```python
from build123d import *

# Parameters (mm, degrees)
IZIM1_W                     = 112.077867903
IZIM1_H                     = 74.551796061
Y_KSEKLIK_EKSTR_ZYON1_DEPTH = 83.934945503
IZIM2_W                     = 101.231343604
IZIM2_H                     = 66.034767048
KES_EKSTR_ZYON2_DEPTH       = 76.644430763
IZIM3_W                     = 39.444954406
IZIM3_H                     = 29.43714267
KES_EKSTR_ZYON3_DEPTH       = 88.138
Y_KSEKLIK_EKSTR_ZYON2_DEPTH = 2.54


with BuildPart() as part:
    # Çizim1 → Yükseklik-Ekstrüzyon1 (new body)
    with BuildSketch(Plane.XY):
        with Locations((-65.092964498, -0.375260719)):
            Rectangle(IZIM1_W, IZIM1_H)
    extrude(amount=Y_KSEKLIK_EKSTR_ZYON1_DEPTH)

    # Çizim2 → Kes-Ekstrüzyon2 (cut)
    with BuildSketch(Plane.XY.offset(83.934945503)):
        with Locations((-64.892181627, -1.311030391)):
            Rectangle(IZIM2_W, IZIM2_H)
    extrude(amount=-KES_EKSTR_ZYON2_DEPTH, mode=Mode.SUBTRACT)

    # Çizim3 → Kes-Ekstrüzyon3 (cut)
    with BuildSketch(Plane.XY.offset(7.29051474)):
        with Locations((-56.533774773, 7.010455604)):
            Rectangle(IZIM3_W, IZIM3_H)
    extrude(amount=-KES_EKSTR_ZYON3_DEPTH, mode=Mode.SUBTRACT)

    # Çizim4 → Yükseklik-Ekstrüzyon2 (add)
    with BuildSketch(Plane(origin=(0, -37.651158749, 0), x_dir=(-1, 0, 0), z_dir=(0, -1, 0))):
        with BuildLine():
            Line((113.611032553, -79.46460314), (113.611032553, -6.689235104))
            ThreePointArc((113.611032553, -6.689235104), (115.960654564, -4.339613094), (118.310276574, -6.689235104))
            Line((118.310276574, -6.689235104), (118.310276574, -79.46460314))
            ThreePointArc((118.310276574, -79.46460314), (115.960654564, -81.814225151), (113.611032553, -79.46460314))
        make_face()
        with BuildLine():
            Line((11.064518037, -78.985150192), (11.064518037, -6.209782156))
            ThreePointArc((11.064518037, -6.209782156), (13.414140048, -3.860160145), (15.763762058, -6.209782156))
            Line((15.763762058, -6.209782156), (15.763762058, -78.985150192))
            ThreePointArc((15.763762058, -78.985150192), (13.414140048, -81.334772203), (11.064518037, -78.985150192))
        make_face()
    extrude(amount=Y_KSEKLIK_EKSTR_ZYON2_DEPTH)


solid = part.part
```
The listing builds one solid part. Answer for the finished solid, in the listing's coordinates (mm). A direction names the side the tool comes from. Coordinates: 2 decimals unless noted, no trailing zeros. Order: outer loops, then holes, each group sorted by start corner. A loop starts at its lowest first (then second) coordinate and runs counter-clockwise, first axis right, second up. Notation, with made-up numbers: M 23,88.25 L 52,88.25 A15 cw 52,114.25 Z; hole C 32,37.25 d11. An arc over 180 degrees is marked long. Answer as a JSON object with one key per item and string values. Group by question number.
1. Section A-A on z = 15.5 is taken. Write down the section's boundary in (x, y), then the cut area to 3 significant figures.
2. A tool of negligible diameter and unlimited length cuts with its end or side. For faces 1 (the flat face through (-15.764, -39, 42)), 2 (the flat face through (-76.256, 7, 4)), 3 (the cylindrical face through (-13.36, -38.9, 3.86)), from which of +Z, -Z, +X, -X, +Y, -Y can it reach the whole face along a straight path? Write none if from no direction.
3. Section B-B on y = 16 is taken. Write down the section's boundary in (x, z).
4. Determine the mould class of faces 4 (the flat face through (-9.054, -1, 41)), 5 (the flat face through (-14.277, -2, 46)), 6 (the flat face through (-121.132, -1, 41)), 7 (the flat face through (-36.811, 7, 4)) for opening direction X: released by +X, released by -X, zero draft, split by the parting line, or undercut.
5. Section C-C on x = -63 is taken. Write down the section's boundary in (y, z).
6. Flat-ended cylindrical pins translate along their axes: P1, Ø2, axis at x = -53, z = 41, coming from the -Y side; P2, Ø0.8, axis at y = -39, z = 41.5, coming from the +X side; P3, Ø0.8, axis at y = -39, z = 33.5, coming from the -X side. Find the tip coordinate at first contact, or state that the pin passes through.
7. Straight lines are drawn through the part: line 1 (Y direction, x = -114, z = 60); line 2 (Y direction, x = -27, z = 80); line 3 (X direction, y = -13, z = 51). For each, find the intervals that lie inside material, in ascending order.
8. Section D-D on y = -20.5 is taken. Write down the section's boundary in (x, z).
Values follow:
{
 "1": {"outline": "M -121.13,-37.65 L -118.31,-37.65 L -118.31,-40.19 L -113.61,-40.19 L -113.61,-37.65 L -15.76,-37.65 L -15.76,-40.19 L -11.06,-40.19 L -11.06,-37.65 L -9.05,-37.65 L -9.05,36.9 L -121.13,36.9 Z; hole M -115.51,-34.33 L -14.28,-34.33 L -14.28,31.71 L -115.51,31.71 Z", "area": "1,690 mm2"},
 "2": {"face 1": "+Z, -Z, -Y", "face 2": "+Z, -Z", "face 3": "-Z, -Y"},
 "3": {"outline": "M -121.13,0 L -76.26,0 L -76.26,7.29 L -115.51,7.29 L -115.51,83.93 L -121.13,83.93 Z; M -36.81,0 L -9.05,0 L -9.05,83.93 L -14.28,83.93 L -14.28,7.29 L -36.81,7.29 Z"},
 "4": {"face 4": "released by +X", "face 5": "undercut", "face 6": "released by -X", "face 7": "undercut"},
 "5": {"outline": "M -37.65,0 L -7.71,0 L -7.71,7.29 L -34.33,7.29 L -34.33,83.93 L -37.65,83.93 Z; M 21.73,0 L 36.9,0 L 36.9,83.93 L 31.71,83.93 L 31.71,7.29 L 21.73,7.29 Z"},
 "6": {"P1": "y = -37.65", "P2": "x = -11.06", "P3": "x = -118.31"},
 "7": {"line 1": "-40.19 to -34.33, 31.71 to 36.9", "line 2": "-37.65 to -34.33, 31.71 to 36.9", "line 3": "-121.13 to -115.51, -14.28 to -9.05"},
 "8": {"outline": "M -121.13,0 L -9.05,0 L -9.05,83.93 L -14.28,83.93 L -14.28,7.29 L -115.51,7.29 L -115.51,83.93 L -121.13,83.93 Z"}
}
